from build123d import *

# Parameters (mm, degrees)
SKETCH1_R           = 4
SKETCH1_R_2         = 1.5
BOSS_EXTRUDE1_DEPTH = 2.5


with BuildPart() as part:
    # Sketch1 → Boss-Extrude1 (new body)
    with BuildSketch(Plane(origin=(0, 0, 0), x_dir=(1, 0, 0), z_dir=(0, 1, 0))):
        with BuildLine():
            ThreePointArc((12.022120265, 67.673247628), (0, 76.75), (-12.022120265, 67.673247628))
            ThreePointArc((-12.022120265, 67.673247628), (-34.842613641, 43.81538777), (-67.414732932, 49.203285306))
            ThreePointArc((-67.414732932, 49.203285306), (-85.189938198, 46.45680917), (-81.819417269, 28.789306741))
            ThreePointArc((-81.819417269, 28.789306741), (-66.25, 0), (-81.819417269, -28.789306741))
            ThreePointArc((-81.819417269, -28.789306741), (-85.189938198, -46.45680917), (-67.414732932, -49.203285306))
            ThreePointArc((-67.414732932, -49.203285306), (-34.842613641, -43.81538777), (-12.022120265, -67.673247628))
            ThreePointArc((-12.022120265, -67.673247628), (0, -76.75), (12.022120265, -67.673247628))
            ThreePointArc((12.022120265, -67.673247628), (34.842613641, -43.81538777), (67.414732932, -49.203285306))
            ThreePointArc((67.414732932, -49.203285306), (85.189938198, -46.45680917), (81.819417269, -28.789306741))
            ThreePointArc((81.819417269, -28.789306741), (66.25, 0), (81.819417269, 28.789306741))
            ThreePointArc((81.819417269, 28.789306741), (85.189938198, 46.45680917), (67.414732932, 49.203285306))
            ThreePointArc((67.414732932, 49.203285306), (34.842613641, 43.81538777), (12.022120265, 67.673247628))
        make_face()
        with Locations(Location((0, 64.25, 0), (0, 0, 270))):
            Circle(SKETCH1_R, mode=Mode.SUBTRACT)
        with Locations(Location((-7, 64.25, 0), (0, 0, 270))):
            Circle(SKETCH1_R_2, mode=Mode.SUBTRACT)
        with Locations(Location((0, 57.25, 0), (0, 0, 270))):
            Circle(SKETCH1_R_2, mode=Mode.SUBTRACT)
        with Locations(Location((7, 64.25, 0), (0, 0, 270))):
            Circle(SKETCH1_R_2, mode=Mode.SUBTRACT)
        with Locations(Location((0, 71.25, 0), (0, 0, 270))):
            Circle(SKETCH1_R_2, mode=Mode.SUBTRACT)
        with Locations(Location((0, 37.375, 0), (0, 0, 270))):
            Circle(SKETCH1_R_2, mode=Mode.SUBTRACT)
        with Locations(Location((17.575, 27.5, 0), (0, 0, 270))):
            Circle(SKETCH1_R_2, mode=Mode.SUBTRACT)
        with Locations(Location((24.9, 37.375, 0), (0, 0, 270))):
            Circle(SKETCH1_R_2, mode=Mode.SUBTRACT)
        with Locations(Location((38.375, 32.75, 0), (0, 0, 270))):
            Circle(SKETCH1_R_2, mode=Mode.SUBTRACT)
        with Locations(Location((47.375, 24.800648389, 0), (0, 0, 270))):
            Circle(SKETCH1_R_2, mode=Mode.SUBTRACT)
        with Locations(Location((74.976618386, 39.25, 0), (0, 0, 270))):
            Circle(SKETCH1_R, mode=Mode.SUBTRACT)
        with Locations(Location((68.775, 36.003474258, 0), (0, 0, 270))):
            Circle(SKETCH1_R_2, mode=Mode.SUBTRACT)
        with Locations(Location((71.730092644, 45.451618386, 0), (0, 0, 270))):
            Circle(SKETCH1_R_2, mode=Mode.SUBTRACT)
        with Locations(Location((81.178236772, 42.496525742, 0), (0, 0, 270))):
            Circle(SKETCH1_R_2, mode=Mode.SUBTRACT)
        with Locations(Location((78.223144128, 33.048381614, 0), (0, 0, 270))):
            Circle(SKETCH1_R_2, mode=Mode.SUBTRACT)
        with Locations(Location((35, 0, 0), (0, 0, 270))):
            Circle(SKETCH1_R_2, mode=Mode.SUBTRACT)
        with Locations(Location((-35, 0, 0), (0, 0, 270))):
            Circle(SKETCH1_R_2, mode=Mode.SUBTRACT)
        with Locations(Location((-47.375, 24.800648389, 0), (0, 0, 270))):
            Circle(SKETCH1_R_2, mode=Mode.SUBTRACT)
        with Locations(Location((-38.375, 32.75, 0), (0, 0, 270))):
            Circle(SKETCH1_R_2, mode=Mode.SUBTRACT)
        with Locations(Location((-17.575, 27.5, 0), (0, 0, 270))):
            Circle(SKETCH1_R_2, mode=Mode.SUBTRACT)
        with Locations(Location((-24.9, 37.375, 0), (0, 0, 270))):
            Circle(SKETCH1_R_2, mode=Mode.SUBTRACT)
        with Locations(Location((-78.223144128, 33.048381614, 0), (0, 0, 270))):
            Circle(SKETCH1_R_2, mode=Mode.SUBTRACT)
        with Locations(Location((-81.178236772, 42.496525742, 0), (0, 0, 270))):
            Circle(SKETCH1_R_2, mode=Mode.SUBTRACT)
        with Locations(Location((-71.730092644, 45.451618386, 0), (0, 0, 270))):
            Circle(SKETCH1_R_2, mode=Mode.SUBTRACT)
        with Locations(Location((-68.775, 36.003474258, 0), (0, 0, 270))):
            Circle(SKETCH1_R_2, mode=Mode.SUBTRACT)
        with Locations(Location((-74.976618386, 39.25, 0), (0, 0, 270))):
            Circle(SKETCH1_R, mode=Mode.SUBTRACT)
        with Locations(Location((-24.9, -37.375, 0), (0, 0, 270))):
            Circle(SKETCH1_R_2, mode=Mode.SUBTRACT)
        with Locations(Location((-17.575, -27.5, 0), (0, 0, 270))):
            Circle(SKETCH1_R_2, mode=Mode.SUBTRACT)
        with Locations(Location((-38.375, -32.75, 0), (0, 0, 270))):
            Circle(SKETCH1_R_2, mode=Mode.SUBTRACT)
        with Locations(Location((-47.375, -24.800648389, 0), (0, 0, 270))):
            Circle(SKETCH1_R_2, mode=Mode.SUBTRACT)
        with Locations(Location((47.375, -24.800648389, 0), (0, 0, 270))):
            Circle(SKETCH1_R_2, mode=Mode.SUBTRACT)
        with Locations(Location((38.375, -32.75, 0), (0, 0, 270))):
            Circle(SKETCH1_R_2, mode=Mode.SUBTRACT)
        with Locations(Location((24.9, -37.375, 0), (0, 0, 270))):
            Circle(SKETCH1_R_2, mode=Mode.SUBTRACT)
        with Locations(Location((17.575, -27.5, 0), (0, 0, 270))):
            Circle(SKETCH1_R_2, mode=Mode.SUBTRACT)
        with Locations(Location((0, -37.375, 0), (0, 0, 270))):
            Circle(SKETCH1_R_2, mode=Mode.SUBTRACT)
        with Locations(Location((0, -71.25, 0), (0, 0, 270))):
            Circle(SKETCH1_R_2, mode=Mode.SUBTRACT)
        with Locations(Location((7, -64.25, 0), (0, 0, 270))):
            Circle(SKETCH1_R_2, mode=Mode.SUBTRACT)
        with Locations(Location((0, -57.25, 0), (0, 0, 270))):
            Circle(SKETCH1_R_2, mode=Mode.SUBTRACT)
        with Locations(Location((-7, -64.25, 0), (0, 0, 270))):
            Circle(SKETCH1_R_2, mode=Mode.SUBTRACT)
        with Locations(Location((0, -64.25, 0), (0, 0, 270))):
            Circle(SKETCH1_R, mode=Mode.SUBTRACT)
        with Locations(Location((78.223144128, -33.048381614, 0), (0, 0, 270))):
            Circle(SKETCH1_R_2, mode=Mode.SUBTRACT)
        with Locations(Location((81.178236772, -42.496525742, 0), (0, 0, 270))):
            Circle(SKETCH1_R_2, mode=Mode.SUBTRACT)
        with Locations(Location((71.730092644, -45.451618386, 0), (0, 0, 270))):
            Circle(SKETCH1_R_2, mode=Mode.SUBTRACT)
        with Locations(Location((68.775, -36.003474258, 0), (0, 0, 270))):
            Circle(SKETCH1_R_2, mode=Mode.SUBTRACT)
        with Locations(Location((74.976618386, -39.25, 0), (0, 0, 270))):
            Circle(SKETCH1_R, mode=Mode.SUBTRACT)
        with Locations(Location((-74.976618386, -39.25, 0), (0, 0, 270))):
            Circle(SKETCH1_R, mode=Mode.SUBTRACT)
        with Locations(Location((-68.775, -36.003474258, 0), (0, 0, 270))):
            Circle(SKETCH1_R_2, mode=Mode.SUBTRACT)
        with Locations(Location((-71.730092644, -45.451618386, 0), (0, 0, 270))):
            Circle(SKETCH1_R_2, mode=Mode.SUBTRACT)
        with Locations(Location((-81.178236772, -42.496525742, 0), (0, 0, 270))):
            Circle(SKETCH1_R_2, mode=Mode.SUBTRACT)
        with Locations(Location((-78.223144128, -33.048381614, 0), (0, 0, 270))):
            Circle(SKETCH1_R_2, mode=Mode.SUBTRACT)
        with Locations(Location((-55.95, 0, 0), (0, 0, 270))):
            Circle(SKETCH1_R_2, mode=Mode.SUBTRACT)
        with Locations(Location((-55.95, 6.875, 0), (0, 0, 270))):
            Circle(SKETCH1_R_2, mode=Mode.SUBTRACT)
        with Locations(Location((-55.95, -6.875, 0), (0, 0, 270))):
            Circle(SKETCH1_R_2, mode=Mode.SUBTRACT)
        with Locations(Location((55.95, 6.875, 0), (0, 0, 270))):
            Circle(SKETCH1_R_2, mode=Mode.SUBTRACT)
        with Locations(Location((55.95, 0, 0), (0, 0, 270))):
            Circle(SKETCH1_R_2, mode=Mode.SUBTRACT)
        with Locations(Location((55.95, -6.875, 0), (0, 0, 270))):
            Circle(SKETCH1_R_2, mode=Mode.SUBTRACT)
        with Locations(Location((0, 0, 0), (0, 0, 270))):
            Circle(SKETCH1_R_2, mode=Mode.SUBTRACT)
    extrude(amount=BOSS_EXTRUDE1_DEPTH)


solid = part.part
Design review of the part built by this model. Coordinates are the model's own, in mm. Coordinates: 2 decimals unless noted, no trailing zeros. Loops run counter-clockwise (first coordinate to the right, second up) from the corner with the lowest first, then second, coordinate; pieces in that order, holes last. Notation, with made-up numbers: (8.5, 25) -> (51.5, 25) arc R15 cw to (51.5, 50) -> close; hole circle Ø3 at (81.5, 83.5). An arc over 180 degrees is marked (long way). Use a Markdown table: item, result. Add a question column.
Item 1: We need section C-C, the plane y = 1.05. Count the separate pieces of the cut face and the enclosed holes in it, and give its area (3 significant figures).
Item 2: We need section B-B, the plane x = -62. Write out the cut boundary in (y, z).
Item 3: We need section A-A, the plane z = 19. Write out the cut boundary in (x, y).
Item 4: Wall thickness on L1, parallel to Z at x = -47.5, y = 1.75; L2, parallel to X at y = 1.2, z = 39; L3, parallel to Z at x = -76.5, y = 1.65: over which ranges is each line inside the solid? List them lowest first. Write a range as from..to.
Item 5: The part is to be moulded in two halves that separate along Z. For faces 1 (the cylindrical face through (85.03, 1.23, 46.68)), 2 (the cylindrical face through (-1.532, 1.232, 67.945)), 3 (the cylindrical face through (-35.3, 1.232, 43.666)), 4 (the cylindrical face through (35.3, 1.232, -43.666)), say which applies: +Z half, -Z half, draft (parallel to the pull), parting line (faces both ways), or undercut.
Item 6: Clearance check with flat-ended pins moving along their axes: P1, Ø4, axis at x = 17.575, z = 27.5, coming from the -Y side; P2, Ø1.5, axis at x = 6.5, y = 0.5, coming from the +Z side; P3, Ø1, axis at x = 64.5, y = 2, coming from the -Z side; P4, Ø1, axis at x = -54.5, y = 1.5, coming from the -Z side. State where each tip first meets the part, or that it passes through.
Numbers:
| question | item | result |
|---|---|---|
| 1 | separate pieces | 1 |
| 1 | enclosed holes | 57 |
| 1 | area | 15,300 mm^2 |
| 2 | outline | (0, -45.81) -> (2.5, -45.81) -> (2.5, 45.81) -> (0, 45.81) -> close |
| 3 | outline | (-71.97, 0) -> (71.97, 0) -> (71.97, 2.5) -> (-71.97, 2.5) -> close |
| 4 | L1 | z = -42.03..-26.3, -23.31..23.31, 26.3..42.03 |
| 4 | L2 | x = -87.47..-78.97, -70.98..70.98, 78.97..87.47 |
| 4 | L3 | z = -51.66..-42.95, -35.55..-24.5, 24.5..35.55, 42.95..51.66 |
| 5 | face 1 | undercut |
| 5 | face 2 | undercut |
| 5 | face 3 | +Z half |
| 5 | face 4 | -Z half |
| 6 | P1 | stops at y = 0 |
| 6 | P2 | stops at z = 75.35 |
| 6 | P3 | stops at z = -47.52 |
| 6 | P4 | stops at z = -43.16 |
